CAD build for the part. Positions are in the model's coordinates, mm. A direction names the side the tool comes from. Give positions to 0.01 mm unless a question says otherwise; leave off trailing zeros. Loops run counter-clockwise (first coordinate to the right, second up) from the corner with the lowest first, then second, coordinate; pieces in that order, holes last.
```python
from build123d import *

# Parameters (mm, degrees)
F0_W     = 101.6
F0_H     = 101.6
F1_DEPTH = 101.6
F2_R     = 25.4
F3_DEPTH = 127.508
F6_W     = 50.8
F6_H     = 50.8
F7_DEPTH = 101.6
F8_R     = 5.08


with BuildPart() as f1:
    # F0 (on Top) → F1 (new body)
    with BuildSketch(Plane.XY):
        Rectangle(F0_W, F0_H)
    extrude(amount=F1_DEPTH)

    # F2 (on face) → F3 (join)
    with BuildSketch(Plane.XY.offset(101.6)):
        Circle(F2_R)
    extrude(amount=F3_DEPTH)

    # F4 (on face) → F5 (revolve)
    with BuildSketch(Plane.XY.offset(229.108)):
        with BuildLine():
            Line((0, -25.4), (0, -38.1))
            ThreePointArc((0, -38.1), (38.1, 0), (0, 38.1))
            Line((0, 38.1), (0, 25.4))
            ThreePointArc((0, 25.4), (17.9605122421, 17.9605122421), (25.4, 0))
            ThreePointArc((25.4, 0), (17.9605122421, -17.9605122421), (0, -25.4))
        make_face()
        with BuildLine():
            ThreePointArc((0, 25.4), (-25.4, 0), (0, -25.4))
            Line((0, -25.4), (0, 25.4))
        make_face()
    revolve(axis=Axis((0, 0, 229.108), (0, -1, 0)))

    # F6 (on face) → F7 (cut)
    with BuildSketch(Plane.XZ.offset(50.8)):
        with Locations((0, 50.8)):
            Rectangle(F6_W, F6_H)
    extrude(amount=-F7_DEPTH, mode=Mode.SUBTRACT)

    # F8
    f8_edges = [f1.edges().sort_by_distance(p)[0] for p in [
        (0, -50.8, 101.6),
        (-50.8, 0, 101.6),
        (50.8, 0, 101.6),
        (0, 50.8, 101.6),
        (50.8, -50.8, 50.8),
        (50.8, 50.8, 50.8),
        (50.8, 0, 0),
        (0, -50.8, 0),
        (-50.8, -50.8, 50.8),
        (-50.8, 50.8, 50.8),
        (-50.8, 0, 0),
        (0, 50.8, 0),
        (-25.4, 0, 200.709937),
        (-25.4, 0, 101.6),
    ]]
    fillet(f8_edges, radius=F8_R)


solid = f1.part
```
1. Drop flat-ended pins along their axis: pin 1 (2 mm diameter, centred on x = 18.5, y = 35, fed in from +Z); pin 2 (4 mm diameter, centred on x = -18, y = -21.5, fed in from +Z); pin 3 (5 mm diameter, centred on y = 26, z = 224, fed in from +X). Give the stop position or say it passes through.
Responses:
pin 1: stops at z = 101.6
pin 2: stops at z = 256.92
pin 3: stops at x = 29.59
2. Pull direction Z, two halves, no side cores. Call faces 4 (the face through (0, -1, 25.4)), 5 (the face through (-1, -50.8, 81)), 6 (the face through (0.64, -49.272, 100.151)): released by +Z, released by -Z, zero draft, split by the parting line, or undercut.
Responses:
face 4: undercut
face 5: zero draft
face 6: released by +Z
3. Saw through at B-B, the plane y = 34. List the corners of the cut face in (x, z).
Responses:
outline: (-50.8, 5.08) arc R5.08 ccw to (-45.72, 0) - (45.72, 0) arc R5.08 ccw to (50.8, 5.08) - (50.8, 96.52) arc R5.08 ccw to (45.72, 101.6) - (-45.72, 101.6) arc R5.08 ccw to (-50.8, 96.52) - close; circle Ø34.39 at (0, 229.11); hole (-25.4, 25.4) - (25.4, 25.4) - (25.4, 76.2) - (-25.4, 76.2) - close
4. Tool access for faces 1 (the face through (49.272, 49.351, 51.44)), 2 (the face through (-25.4, -1, 50)), 3 (the face through (-1, 31, 101.6)): list every direction of +Z, -Z, +X, -X, +Y, -Y with a clear straight run to the whole face (end or side of a thin tool).
Responses:
face 1: +Z, -Z, +X, +Y
face 2: +Y, -Y
face 3: none
5. Saw through at A-A, the plane z = 50.5. List the corners of the cut face in (x, y).
Responses:
outline: (-50.8, -45.72) arc R5.08 ccw to (-45.72, -50.8) - (-25.4, -50.8) - (-25.4, 50.8) - (-45.72, 50.8) arc R5.08 ccw to (-50.8, 45.72) - close; (25.4, -50.8) - (45.72, -50.8) arc R5.08 ccw to (50.8, -45.72) - (50.8, 45.72) arc R5.08 ccw to (45.72, 50.8) - (25.4, 50.8) - close
6. Saw through at C-C, the plane x = 43. List the corners of the cut face in (y, z), and give its area (3 significant figures).
Responses:
outline: (-50.8, 5.08) arc R5.08 ccw to (-45.72, 0) - (45.72, 0) arc R5.08 ccw to (50.8, 5.08) - (50.8, 96.52) arc R5.08 ccw to (45.72, 101.6) - (-45.72, 101.6) arc R5.08 ccw to (-50.8, 96.52) - close
area: 10,300 mm2
7. Probe line 1 along X through (y, z) = (37, 64); line 2 along Z through (x, y) = (11.5, -38); line 3 along Z through (x, y) = (-21, 26.5). List the from-to ranges inside material, lowest first.
Responses:
line 1: x = -50.8 to -25.4, 25.4 to 50.8
line 2: z = 0 to 25.4, 76.2 to 101.6
line 3: z = 0 to 25.4, 76.2 to 101.6, 211.55 to 246.67
8. Saw through at D-D, the plane z = 250. List the corners of the cut face in (x, y).
Responses:
outline: circle Ø63.72 at (0, 0)
